Build history of the part. All positions in model axes, mm. A direction names the side the tool comes from. Give positions to 0.01 mm unless a question says otherwise; leave off trailing zeros. Write each loop counter-clockwise with the first axis right and the second up, starting at its lowest first coordinate (ties: lowest second). Pieces come first, ordered by that corner, then holes.
from build123d import *

# Parameters (mm, degrees)
SKETCH1_W            = 91.936945468
SKETCH1_H            = 61.663418702
SKETCH1_W_2          = 86.36
SKETCH1_H_2          = 56.134
BOSS_EXTRUDE1_DEPTH  = 20
SKETCH2_W            = 86.36
SKETCH2_H            = 56.134
BOSS_EXTRUDE3_DEPTH  = 1
SKETCH4_W            = 80
SKETCH4_H            = 53.28
CUT_EXTRUDE6_DEPTH   = 59.853162931
SKETCH5_W            = 155.947075919
SKETCH5_H            = 20
BOSS_EXTRUDE4_DEPTH  = 3
SKETCH8_W            = 12.917881336
SKETCH8_H            = 3
CUT_EXTRUDE7_DEPTH   = 88.335862802
SKETCH9_W            = 12.878183793
SKETCH9_H            = 3
CUT_EXTRUDE8_DEPTH   = 88.300413605
SKETCH10_R           = 2
CUT_EXTRUDE9_DEPTH   = 94.894510599
SKETCH10_3_R         = 2
CUT_EXTRUDE10_DEPTH  = 94.894510599
SKETCH11_W           = 74.933585118
SKETCH11_H           = 15.731166257
CUT_EXTRUDE11_DEPTH  = 20
FILLET1_R            = 2.54
FILLET2_R            = 2.54
FILLET3_R            = 2.54
FILLET4_R            = 2.54
FILLET5_R            = 2.54
FILLET6_R            = 2.54
SKETCH14_W           = 5.713207441
SKETCH14_H           = 8.255
CUT_EXTRUDE12_DEPTH  = 91.021549452
SKETCH15_W           = 5.713207441
SKETCH15_H           = 8.255
CUT_EXTRUDE13_DEPTH  = 91.021549452
SKETCH16_W           = 7.476166257
SKETCH16_H           = 6.35
BOSS_EXTRUDE5_DEPTH  = 5.713207
SKETCH17_W           = 7.476166257
SKETCH17_H           = 6.35
BOSS_EXTRUDE6_DEPTH  = 5.713207441
SKETCH18_W           = 11.38
SKETCH18_H           = 10.16
BOSS_EXTRUDE7_DEPTH  = 5.713207441
SKETCH19_W           = 11.38
SKETCH19_H           = 10.16
BOSS_EXTRUDE8_DEPTH  = 5.713207441
SKETCH20_W           = 71.616945468
SKETCH20_H           = 9.886340198
CUT_EXTRUDE14_DEPTH  = 94.894510599
SKETCH23_W           = 130.15101079
SKETCH23_H           = 3
BOSS_EXTRUDE14_DEPTH = 2.54


with BuildPart() as part:
    # Sketch1 → Boss-Extrude1 (new body)
    with BuildSketch(Plane.XY):
        Rectangle(SKETCH1_W, SKETCH1_H)
        Rectangle(SKETCH1_W_2, SKETCH1_H_2, mode=Mode.SUBTRACT)
    extrude(amount=BOSS_EXTRUDE1_DEPTH)

    # Sketch2 → Boss-Extrude3 (add)
    with BuildSketch(Plane.XY.offset(20)):
        Rectangle(SKETCH2_W, SKETCH2_H)
    extrude(amount=-BOSS_EXTRUDE3_DEPTH)

    # Sketch4 → Cut-Extrude6 (cut, through all)
    with BuildSketch(Plane.XY.offset(20)):
        Rectangle(SKETCH4_W, SKETCH4_H)
    extrude(amount=-CUT_EXTRUDE6_DEPTH, mode=Mode.SUBTRACT)

    # Sketch5 → Boss-Extrude4 (add)
    with BuildSketch(Plane(origin=(0, 30.831709351, 0), x_dir=(1, 0, 0), z_dir=(0, 1, 0))):
        with Locations((0.019848772, -10)):
            Rectangle(SKETCH5_W, SKETCH5_H)
    extrude(amount=BOSS_EXTRUDE4_DEPTH)

    # Sketch8 → Cut-Extrude7 (cut, through all)
    with BuildSketch(Plane.XY.offset(20)):
        with Locations((71.534446063, 32.331709351)):
            Rectangle(SKETCH8_W, SKETCH8_H)
    extrude(amount=-CUT_EXTRUDE7_DEPTH, mode=Mode.SUBTRACT)

    # Sketch9 → Cut-Extrude8 (cut, through all)
    with BuildSketch(Plane.XY.offset(20)):
        with Locations((-71.514597291, 32.331709351)):
            Rectangle(SKETCH9_W, SKETCH9_H)
    extrude(amount=-CUT_EXTRUDE8_DEPTH, mode=Mode.SUBTRACT)

    # Sketch10 → Cut-Extrude9 (cut, through all)
    with BuildSketch(Plane(origin=(0, 33.831709351, 0), x_dir=(1, 0, 0), z_dir=(0, 1, 0))):
        with Locations(Location((53.249133704, -11, 0), (0, 0, 270))):
            Circle(SKETCH10_R)
    extrude(amount=-CUT_EXTRUDE9_DEPTH, mode=Mode.SUBTRACT)

    # Sketch10<3> → Cut-Extrude10 (cut, through all)
    with BuildSketch(Plane(origin=(0, 33.831709351, 0), x_dir=(1, 0, 0), z_dir=(0, 1, 0))):
        with Locations(Location((53.249133704, -11, 0), (0, 0, 270))):
            Circle(SKETCH10_3_R)
        with Locations(Location((-51.881510593, -11, 0), (0, 0, 270))):
            Circle(SKETCH10_3_R)
    extrude(amount=-CUT_EXTRUDE10_DEPTH, mode=Mode.SUBTRACT)

    # Sketch11 → Cut-Extrude11 (cut)
    with BuildSketch(Plane(origin=(0, 33.831709351, 0), x_dir=(1, 0, 0), z_dir=(0, 1, 0))):
        with Locations((0, -7.865583129)):
            Rectangle(SKETCH11_W, SKETCH11_H)
    extrude(amount=-CUT_EXTRUDE11_DEPTH, mode=Mode.SUBTRACT)

    # Fillet1
    fillet1_edges = [part.edges().sort_by_distance(p)[0] for p in [
        (40, 26.64, 19.5),
    ]]
    fillet(fillet1_edges, radius=FILLET1_R)

    # Fillet2
    fillet2_edges = [part.edges().sort_by_distance(p)[0] for p in [
        (-40, 26.64, 19.5),
    ]]
    fillet(fillet2_edges, radius=FILLET2_R)

    # Fillet3
    fillet3_edges = [part.edges().sort_by_distance(p)[0] for p in [
        (-40, -26.64, 19.5),
    ]]
    fillet(fillet3_edges, radius=FILLET3_R)

    # Fillet4
    fillet4_edges = [part.edges().sort_by_distance(p)[0] for p in [
        (40, -26.64, 19.5),
    ]]
    fillet(fillet4_edges, radius=FILLET4_R)

    # Fillet5
    fillet5_edges = [part.edges().sort_by_distance(p)[0] for p in [
        (-45.968472734, -30.831709351, 10),
    ]]
    fillet(fillet5_edges, radius=FILLET5_R)

    # Fillet6
    fillet6_edges = [part.edges().sort_by_distance(p)[0] for p in [
        (45.968472734, -30.831709351, 10),
    ]]
    fillet(fillet6_edges, radius=FILLET6_R)

    # Sketch14 → Cut-Extrude12 (cut, through all)
    with BuildSketch(Plane.XZ.offset(-28.067)):
        with Locations((40.32339628, 11.603666257)):
            Rectangle(SKETCH14_W, SKETCH14_H)
    extrude(amount=-CUT_EXTRUDE12_DEPTH, mode=Mode.SUBTRACT)

    # Sketch15 → Cut-Extrude13 (cut, through all)
    with BuildSketch(Plane.XZ.offset(-28.067)):
        with Locations((-40.32339628, 11.603666257)):
            Rectangle(SKETCH15_W, SKETCH15_H)
    extrude(amount=-CUT_EXTRUDE13_DEPTH, mode=Mode.SUBTRACT)

    # Sketch16 → Boss-Extrude5 (add)
    with BuildSketch(Plane.ZY.offset(-43.18)):
        with Locations((3.738083129, 24.892)):
            Rectangle(SKETCH16_W, SKETCH16_H)
    extrude(amount=BOSS_EXTRUDE5_DEPTH)

    # Sketch17 → Boss-Extrude6 (add)
    with BuildSketch(Plane(origin=(-43.18, 0, 0), x_dir=(0, 0, -1), z_dir=(1, 0, 0))):
        with Locations((-3.738083129, 24.892)):
            Rectangle(SKETCH17_W, SKETCH17_H)
    extrude(amount=BOSS_EXTRUDE6_DEPTH)

    # Sketch18 → Boss-Extrude7 (add)
    with BuildSketch(Plane(origin=(-43.18, 0, 0), x_dir=(0, 0, -1), z_dir=(1, 0, 0))):
        with Locations((-5.69, -22.987)):
            Rectangle(SKETCH18_W, SKETCH18_H)
    extrude(amount=BOSS_EXTRUDE7_DEPTH)

    # Sketch19 → Boss-Extrude8 (add)
    with BuildSketch(Plane.ZY.offset(-43.18)):
        with Locations((5.69, -22.987)):
            Rectangle(SKETCH19_W, SKETCH19_H)
    extrude(amount=BOSS_EXTRUDE8_DEPTH)

    # Sketch20 → Cut-Extrude14 (cut, through all)
    with BuildSketch(Plane.XZ.offset(30.831709351)):
        with Locations((0, 4.943170099)):
            Rectangle(SKETCH20_W, SKETCH20_H)
    extrude(amount=-CUT_EXTRUDE14_DEPTH, mode=Mode.SUBTRACT)

    # Sketch23 → Boss-Extrude14 (add)
    # profile 1 of 2: a face of its own
    with BuildSketch(Plane.XY.offset(20)):
        with BuildLine():
            Line((-43.428472734, -30.831709351), (43.428472734, -30.831709351))
            ThreePointArc((43.428472734, -30.831709351), (45.224523958, -30.087760575), (45.968472734, -28.291709351))
            Line((45.968472734, -28.291709351), (45.968472734, 30.831709351))
            Line((45.968472734, 30.831709351), (-45.968472734, 30.831709351))
            Line((-45.968472734, 30.831709351), (-45.968472734, -28.291709351))
            ThreePointArc((-45.968472734, -28.291709351), (-45.224523958, -30.087760575), (-43.428472734, -30.831709351))
        make_face()
        with BuildLine():
            ThreePointArc((39.537823304, -25.560907361), (38.61351341, -26.44781055), (37.373915264, -26.770831426))
            Line((37.373915264, -26.770831426), (-37.373915264, -26.770831426))
            ThreePointArc((-37.373915264, -26.770831426), (-38.61351341, -26.44781055), (-39.537823304, -25.560907361))
            ThreePointArc((-39.537823304, -25.560907361), (-39.881700972, -24.866136022), (-40, -24.1))
            Line((-40, -24.1), (-40, 24.1))
            ThreePointArc((-40, 24.1), (-39.881700972, 24.866136022), (-39.537823304, 25.560907361))
            ThreePointArc((-39.537823304, 25.560907361), (-38.61351341, 26.44781055), (-37.373915264, 26.770831426))
            Line((-37.373915264, 26.770831426), (37.373915264, 26.770831426))
            ThreePointArc((37.373915264, 26.770831426), (38.61351341, 26.44781055), (39.537823304, 25.560907361))
            ThreePointArc((39.537823304, 25.560907361), (39.881700972, 24.866136022), (40, 24.1))
            Line((40, 24.1), (40, -24.1))
            ThreePointArc((40, -24.1), (39.881700972, -24.866136022), (39.537823304, -25.560907361))
        make_face(mode=Mode.SUBTRACT)
    # profile 2 of 2: a face of its own
    with BuildSketch(Plane.XY.offset(20)):
        with Locations((0, 32.331709351)):
            Rectangle(SKETCH23_W, SKETCH23_H)
    extrude(amount=BOSS_EXTRUDE14_DEPTH)


solid = part.part
(1) Saw through at A-A, the plane y = -12. List the corners of the cut face in (x, z), plus the area to 3 significant figures.
(2) Mould opens along X. For faces 1 (the face through (-1, 31, 15.731)), 2 (the face through (-1, 33.832, 16)) say: +X half, -X half, draft (parallel to the pull), parting line (faces both ways), or undercut.
(3) Saw through at C-C, the plane z = 4. List the corners of the cut face in (x, y).
(4) Saw through at B-B, the plane x = -1. List the corners of the cut face in (y, z).
(5) 3-axis set-ups, long thin cutter, end or side, ignore diameter. For faces 3 (the face through (-43.18, 2, 11)), 4 (the face through (-40, 21.717, 4)), 5 (the face through (40, -23, 11.38)), 6 (the face through (-1, -29, 9.886)): which of +Z, -Z, +X, -X, +Y, -Y reach the whole face in a straight line?
(6) Drop flat-ended pins along their axis: pin 1 (7 mm diameter, centred on y = -5.5, z = 14, fed in from -X); pin 2 (4 mm diameter, centred on x = -49, y = 15.5, fed in from -Z); pin 3 (4.5 mm diameter, centred on x = -51.88, z = 11, fed in from -Y); pin 4 (12 mm diameter, centred on x = -15.5, z = 8, fed in from +Y). Give the stop position or say it passes through.
(7) Probe line 1 (X direction, y = 32.65, z = 11); line 2 (Y direction, x = -21, z = 18.75); line 3 (X direction, y = -7, z = 18.75). List the from-to ranges inside material, lowest first.
Computed values:
1. outline: (-45.97, 0) - (-43.18, 0) - (-43.18, 19) - (-40, 19) - (-40, 22.54) - (-45.97, 22.54) - close; (40, 19) - (43.18, 19) - (43.18, 0) - (45.97, 0) - (45.97, 22.54) - (40, 22.54) - close
1. area: 148 mm2
2. face 1: undercut
2. face 2: draft
3. outline: (-65.08, 30.83) - (-45.97, 30.83) - (-45.97, -28.29) arc R2.54 ccw to (-43.43, -30.83) - (-35.81, -30.83) - (-35.81, -28.07) - (-37.47, -28.07) - (-37.47, -17.91) - (-43.18, -17.91) - (-43.18, 21.72) - (-37.47, 21.72) - (-37.47, 33.83) - (-65.08, 33.83) - close; (35.81, -30.83) - (43.43, -30.83) arc R2.54 ccw to (45.97, -28.29) - (45.97, 30.83) - (65.08, 30.83) - (65.08, 33.83) - (37.47, 33.83) - (37.47, 21.72) - (43.18, 21.72) - (43.18, -17.91) - (37.47, -17.91) - (37.47, -28.07) - (35.81, -28.07) - close
4. outline: (-30.83, 9.89) - (-28.07, 9.89) - (-28.07, 19) - (-26.64, 19) - (-26.64, 20) - (-26.77, 20) - (-26.77, 22.54) - (-30.83, 22.54) - close; (26.64, 19) - (28.07, 19) - (28.07, 15.73) - (33.83, 15.73) - (33.83, 22.54) - (26.77, 22.54) - (26.77, 20) - (26.64, 20) - close
5. face 3: none
5. face 4: -Z
5. face 5: +Y
5. face 6: -Z, +Y, -Y
6. pin 1: stops at x = -45.97
6. pin 2: passes through
6. pin 3: stops at y = 30.83
6. pin 4: stops at y = -28.07
7. line 1: x = -65.08 to -53.88, -49.88 to -43.18, 43.18 to 51.25, 55.25 to 65.08
7. line 2: y = -30.83 to -28.07, 28.07 to 33.83
7. line 3: x = -45.97 to -43.18, 43.18 to 45.97
